Can you work these out from the model? Positions are in its coordinate system, mm. A direction names the side the tool comes from. Round coordinates to 2 decimals unless told otherwise and drop trailing zeros. Write each loop counter-clockwise with the first axis right and the second up, starting at its lowest first coordinate (ties: lowest second). Pieces come first, ordered by that corner, then holes. Notation, with made-up numbers: M -6,-9 L 0,-9 A22 cw 0,19 Z; hole C -22,35 d3. An arc over 180 degrees is marked long. Answer in a Markdown table with one row per item. Add a question column.
(1) I'm going to push flat-ended pins straight in: pin 1 (2 mm diameter, centred on x = -23, y = -44, fed in from +Z); pin 2 (10 mm diameter, centred on x = 29.5, y = -31, fed in from +Z). Where does each tip first touch, or does it pass through?
(2) If we mould it in two halves opening along Y, with no side actions, what happens to faces 1 (the face through (0.98, -139.01, -74.53)), 2 (the face through (-48.46, -26.93, 25.35)), 3 (the face through (-1, -69, -76.055))? For each: released by +Y, released by -Y, zero draft, split by the parting line, or undercut.
(3) Suppose I cut it at B-B, the plane y = -60. Write out the boundary of the cut face in (x, z), then the cut area to 3 significant figures.
(4) If I drill on probe 1 along Y at (x, z) = (38.5, 48); probe 2 along X at (y, z) = (-95.5, -3.5); probe 3 along Z at (x, y) = (-24.5, -93), over which ranges is the centre line in solid material (lowest first)?
(5) Suppose I cut it at A-A, the plane z = 10. Write out the boundary of the cut face in (x, y), then the cut area to 3 significant figures.
(6) For faces 4 (the face through (-1, -115.062, 25)), 5 (the face through (73.78, -71.14, 73.24)), which set-ups out of +Z, -Z, +X, -X, +Y, -Y let a thin tool reach every point of the face, with its end or its side?
(7) Suppose I cut it at C-C, the plane x = 13.5. Write out the boundary of the cut face in (y, z).
from build123d import *

# Parameters (mm, degrees)
F0_W     = 150.6082415581
F0_H     = 150.7464423776
F1_DEPTH = 140.462
F2_T     = -25.4
F3_DEPTH = 25.4
F5_R     = 5.08


with BuildPart() as f1:
    # F0 (on Front) → F1 (new body)
    with BuildSketch(Plane.XZ):
        with Locations((0, -0.6814859807)):
            Rectangle(F0_W, F0_H)
    extrude(amount=F1_DEPTH)

    # F2
    f2_openings = [f1.faces().sort_by_distance(p)[0] for p in [
        (0, -70.231, 74.691735),
    ]]
    offset(amount=F2_T, openings=f2_openings)

    # F3 (add): a face of the model
    f3_faces = [f1.faces().sort_by_distance(p)[0] for p in [
        (0, -70.231, -50.6547071695),
    ]]
    extrude(f3_faces, amount=F3_DEPTH)

    # F5
    f5_edges = [f1.edges().sort_by_distance(p)[0] for p in [
        (0, -25.4, -25.254707),
        (49.904121, -70.231, -25.254707),
        (-49.904121, -70.231, -25.254707),
        (0, -115.062, -25.254707),
        (0, 0, 74.691735),
        (75.304121, -70.231, 74.691735),
        (0, -140.462, 74.691735),
        (-75.304121, -70.231, 74.691735),
        (49.904121, -70.231, 74.691735),
        (0, -25.4, 74.691735),
        (-49.904121, -70.231, 74.691735),
        (0, -115.062, 74.691735),
        (-75.304121, -70.231, -76.054707),
        (75.304121, -70.231, -76.054707),
        (0, 0, -76.054707),
        (0, -140.462, -76.054707),
        (-75.304121, -140.462, -0.681486),
        (75.304121, -140.462, -0.681486),
        (75.304121, 0, -0.681486),
        (-75.304121, 0, -0.681486),
        (-49.904121, -25.4, 24.718514),
        (-49.904121, -115.062, 24.718514),
        (49.904121, -115.062, 24.718514),
        (49.904121, -25.4, 24.718514),
    ]]
    fillet(f5_edges, radius=F5_R)


solid = f1.part
Calculated:
| question | item | result |
|---|---|---|
| 1 | pin 1 | z = -25.25 |
| 1 | pin 2 | z = -22.57 |
| 2 | face 1 | released by -Y |
| 2 | face 2 | undercut |
| 2 | face 3 | zero draft |
| 3 | outline | M -75.3,-70.97 A5.08 ccw -70.22,-76.05 L 70.22,-76.05 A5.08 ccw 75.3,-70.97 L 75.3,69.61 A5.08 ccw 70.22,74.69 L 54.98,74.69 A5.08 ccw 49.9,69.61 L 49.9,-20.17 A5.08 cw 44.82,-25.25 L -44.82,-25.25 A5.08 cw -49.9,-20.17 L -49.9,69.61 A5.08 ccw -54.98,74.69 L -70.22,74.69 A5.08 ccw -75.3,69.61 Z |
| 3 | area | 12,700 mm² |
| 4 | probe 1 | -140.46 to -115.06, -25.4 to 0 |
| 4 | probe 2 | -75.3 to -49.9, 49.9 to 75.3 |
| 4 | probe 3 | -76.05 to -25.25 |
| 5 | outline | M -75.3,-135.38 A5.08 ccw -70.22,-140.46 L 70.22,-140.46 A5.08 ccw 75.3,-135.38 L 75.3,-5.08 A5.08 ccw 70.22,0 L -70.22,0 A5.08 ccw -75.3,-5.08 Z; hole M -49.9,-109.98 A5.08 ccw -44.82,-115.06 L 44.82,-115.06 A5.08 ccw 49.9,-109.98 L 49.9,-30.48 A5.08 ccw 44.82,-25.4 L -44.82,-25.4 A5.08 ccw -49.9,-30.48 Z |
| 5 | area | 12,200 mm² |
| 6 | face 4 | +Z |
| 6 | face 5 | +Z, +X, +Y, -Y |
| 7 | outline | M -140.46,-70.97 A5.08 ccw -135.38,-76.05 L -5.08,-76.05 A5.08 ccw 0,-70.97 L 0,69.61 A5.08 ccw -5.08,74.69 L -20.32,74.69 A5.08 ccw -25.4,69.61 L -25.4,-20.17 A5.08 cw -30.48,-25.25 L -109.98,-25.25 A5.08 cw -115.06,-20.17 L -115.06,69.61 A5.08 ccw -120.14,74.69 L -135.38,74.69 A5.08 ccw -140.46,69.61 Z |
